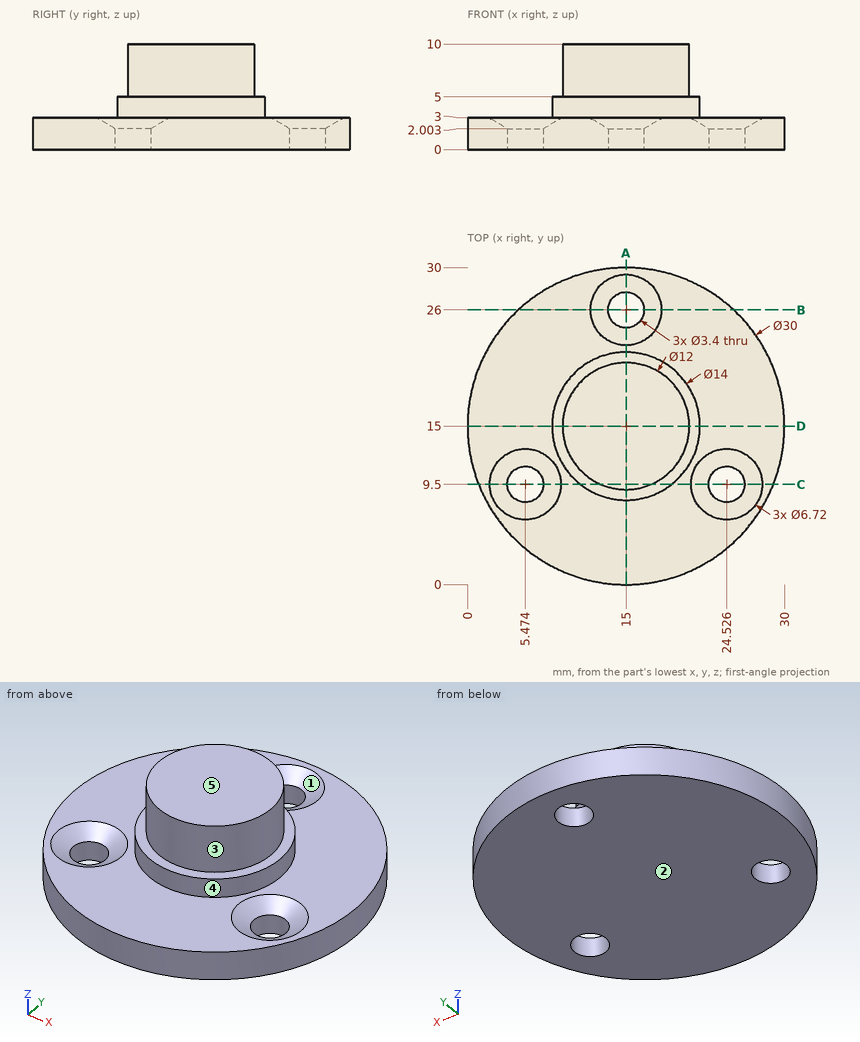
Print and shaded views of the part. All mm, measured from the part's lowest x, y and z. A direction names the side the tool comes from. Round coordinates to 2 decimals unless told otherwise and drop trailing zeros. Write each loop counter-clockwise with the first axis right and the second up, starting at its lowest first coordinate (ties: lowest second). Pieces come first, ordered by that corner, then holes.
(1) Probe line 1 along Y through (x, z) = (15, 1.25); line 2 along X through (y, z) = (9.5, 0.55) (1 decimal); line 3 along Z through (x, y) = (8.5, 21.25). List the from-to ranges inside material, lowest first.
(2) Slice it at D-D, the plane y = 15. Write the cut outline in (x, z), and give its area (3 significant figures).
(3) Drop flat-ended pins along their axis: P1, Ø4, axis at x = 24.53, y = 9.5, coming from the +Z side (1 decimal); P2, Ø5, axis at x = 12.5, z = 7, coming from the -Y side; P3, Ø3, axis at y = 7.5, z = 1.5, coming from the -X side. Give the stop position or say it passes through.
(4) Slice it at C-C, the plane y = 9.5. Write the cut outline in (x, z) (1 decimal).
(5) Slice it at A-A, the plane x = 15. Write the cut outline in (y, z), and give its area (3 significant figures).
(6) Slice it at B-B, the plane y = 26. Write the cut outline in (x, z).
(7) 3-axis set-ups, long thin cutter, end or side, ignore diameter. For the marked faces 4 and 5: which of +Z, -Z, +X, -X, +Y, -Y reach the whole face in a straight line?
(8) Mould opens along Y. For the marked faces 1, 2 and 3 say: pulls with the +Y half, pulls with the -Y half, needs draft (parallel to the pull), parting line crosses it, or undercut.
From the geometry:
1. line 1: y = 0 to 24.3, 27.7 to 30
1. line 2: x = 1 to 3.8, 7.2 to 22.8, 26.2 to 29
1. line 3: z = 0 to 3
2. outline: (0, 0) - (30, 0) - (30, 3) - (22, 3) - (22, 5) - (21, 5) - (21, 10) - (9, 10) - (9, 5) - (8, 5) - (8, 3) - (0, 3) - close
2. area: 178 mm2
3. P1: stops at z = 2.2
3. P2: stops at y = 8.07
3. P3: stops at x = 1.25
4. outline: (1, 0) - (3.8, 0) - (3.8, 2) - (2.1, 3) - (1, 3) - close; (7.2, 0) - (22.8, 0) - (22.8, 2) - (21.2, 3) - (19.3, 3) - (19.3, 5) - (17.4, 5) - (17.4, 10) - (12.6, 10) - (12.6, 5) - (10.7, 5) - (10.7, 3) - (8.8, 3) - (7.2, 2) - close; (26.2, 0) - (29, 0) - (29, 3) - (27.9, 3) - (26.2, 2) - close
5. outline: (0, 0) - (24.3, 0) - (24.3, 2) - (22.64, 3) - (22, 3) - (22, 5) - (21, 5) - (21, 10) - (9, 10) - (9, 5) - (8, 5) - (8, 3) - (0, 3) - close; (27.7, 0) - (30, 0) - (30, 3) - (29.36, 3) - (27.7, 2) - close
5. area: 166 mm2
6. outline: (4.8, 0) - (13.3, 0) - (13.3, 2) - (11.64, 3) - (4.8, 3) - close; (16.7, 0) - (25.2, 0) - (25.2, 3) - (18.36, 3) - (16.7, 2) - close
7. face 4: +Z
7. face 5: +Z, +X, -X, +Y, -Y
8. face 1: undercut
8. face 2: needs draft
8. face 3: parting line crosses it
